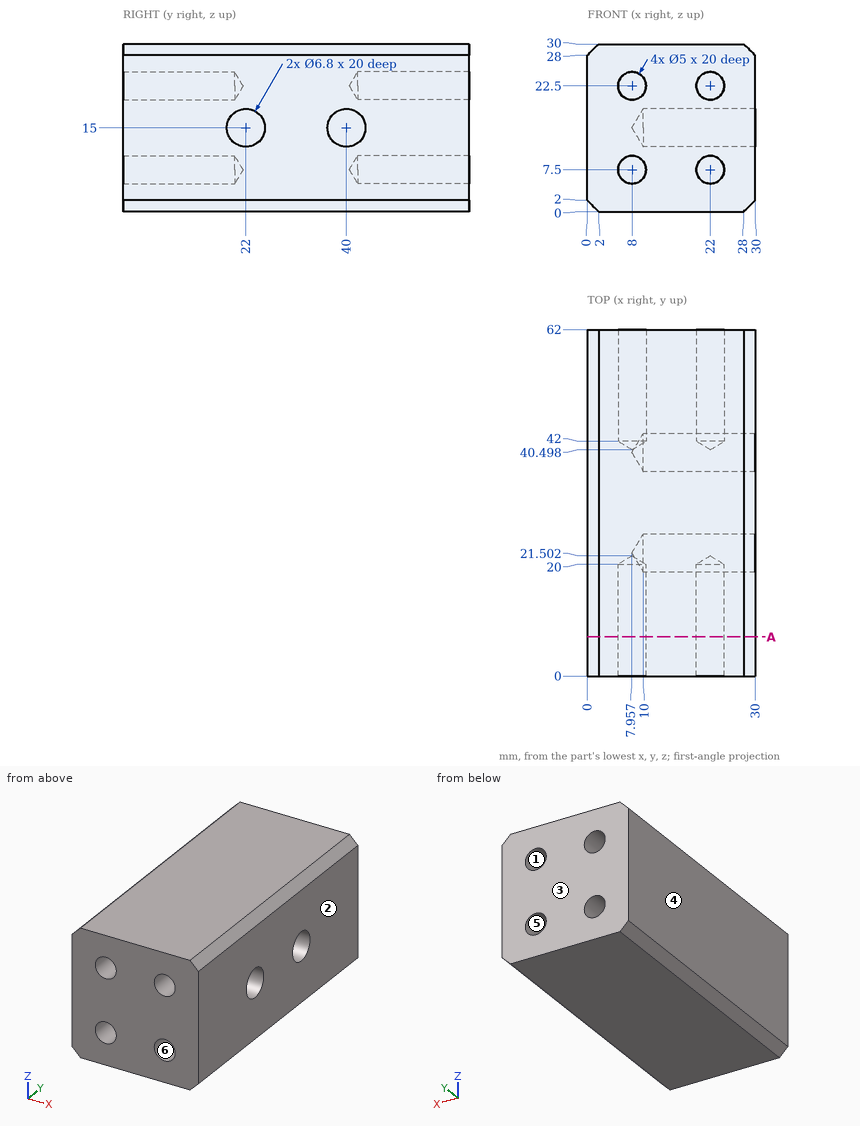
Design review of the part shown in the three views and the two pictorial views. Dimensions are in mm from the part's minimum x, y and z. A direction names the side the tool comes from. Round coordinates to 2 decimals unless told otherwise and drop trailing zeros. Loops run counter-clockwise (first coordinate to the right, second up) from the corner with the lowest first, then second, coordinate; pieces in that order, holes last. Notation, with made-up numbers: M 58,0 L 111,0 A11 ccw 111,19 Z; hole C -26,-26.75 d9. An arc over 180 degrees is marked long. Answer as a JSON object with one key per item and string values.
Item 1: Tool access review of the marked faces 4, 5 and 6: name each direction out of +Z, -Z, +X, -X, +Y, -Y from which nothing blocks a thin tool from reaching the whole face with its end or side.
Check sheet entries:
{"face 4": "+Z, -Z, -X, +Y, -Y", "face 5": "+Y", "face 6": "-Y"}
Item 2: Clearance check with flat-ended pins moving along their axes: P1, Ø3, axis at x = 8, z = 22.5, coming from the +Y side; P2, Ø3, axis at x = 8, z = 22.5, coming from the -Y side; P3, Ø4.5, axis at x = 8, z = 7.5, coming from the -Y side. State where each tip first meets the part, or that it passes through.
Check sheet entries:
{"P1": "y = 41.4", "P2": "y = 20.6", "P3": "y = 20.15"}
Item 3: We need section A-A, the plane y = 7. State the section outline as (x, z) points.
Check sheet entries:
{"outline": "M 0,2 L 2,0 L 28,0 L 30,2 L 30,28 L 28,30 L 2,30 L 0,28 Z; hole C 8,7.5 d5; hole C 8,22.5 d5; hole C 22,7.5 d5; hole C 22,22.5 d5"}
Item 4: The part is to be moulded in two halves that separate along X. For the marked faces 1, 2 and 3, say which applies: +X half, -X half, draft (parallel to the pull), parting line (faces both ways), or undercut.
Check sheet entries:
{"face 1": "undercut", "face 2": "+X half", "face 3": "draft"}
Item 5: For line 1 along X through (y, z) = (55.5, 22.5); line 2 along Y through (x, z) = (20.25, 15); line 3 along Z through (x, y) = (18, 40), list the stretches that pass through material, from the lowest coordinate up.
Check sheet entries:
{"line 1": "0 to 5.5, 10.5 to 19.5, 24.5 to 30", "line 2": "0 to 18.6, 25.4 to 36.6, 43.4 to 62", "line 3": "0 to 11.6, 18.4 to 30"}
